```python
from build123d import *

# Parameters (mm, degrees)
F1_DEPTH    = 5
F2_T1_DEPTH = 21.2627511202


# Not quite as in the source:
# - a fillet or chamfer that OpenCascade refuses, or shapes differently, is made with other operations: its cross-section is extruded or revolved along the edge and cut away or added


with BuildPart() as f1:
    # F0 (on Front) → F1 (new body)
    with BuildSketch(Plane.XZ):
        with BuildLine():
            Line((4, -0.5), (5, -0.5))
            ThreePointArc((5, -0.5), (4.7071067812, 0.2071067812), (4, 0.5))
            Line((4, 0.5), (-4, 0.5))
            ThreePointArc((-4, 0.5), (-4.7071067812, 0.2071067812), (-5, -0.5))
            Line((-5, -0.5), (-4, -0.5))
            ThreePointArc((-4, -0.5), (-3.2187502413, -1.2763021336), (-3.625, -2.3))
            Line((-3.625, -2.3), (-2.75, -6.5))
            Line((-2.75, -6.5), (0, -6.5))
            Line((0, -6.5), (2.75, -6.5))
            Line((2.75, -6.5), (3.625, -2.3))
            ThreePointArc((3.625, -2.3), (3.2187502413, -1.2763021336), (4, -0.5))
        make_face()
    extrude(amount=F1_DEPTH)

    # F2: fillet of radius 4 on 2 edges, made by hand

    # F2_s2 → F2_t1 (cut)
    with BuildSketch(Plane.XZ.offset(-8.1313755601)):
        with BuildLine():
            ThreePointArc((0.502550224, -6.5), (-2.0210119343, -5.6034873985), (-3.4133714549, -3.3158170164))
            Line((-3.4133714549, -3.3158170164), (-2.75, -6.5))
            Line((-2.75, -6.5), (0.502550224, -6.5))
        make_face()
        with BuildLine():
            ThreePointArc((3.4133714549, -3.3158170164), (2.0210119343, -5.6034873985), (-0.502550224, -6.5))
            Line((-0.502550224, -6.5), (2.75, -6.5))
            Line((2.75, -6.5), (3.4133714549, -3.3158170164))
        make_face()
    extrude(amount=F2_T1_DEPTH, mode=Mode.SUBTRACT)


solid = f1.part
```
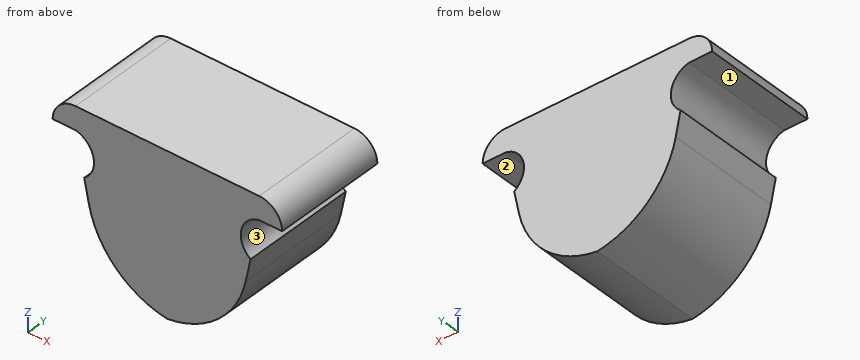
Input: part model. Units: mm. Frame: model coordinates. Face numbers are marked on the shaded views. A direction names the side the tool comes from. Give positions to 0.01 mm unless a question says otherwise; leave off trailing zeros. Order: outer loops, then holes, each group sorted by start corner. A loop starts at its lowest first (then second) coordinate and runs counter-clockwise, first axis right, second up.
1. Section B-B on x = -3. Return the cut outline in (y, z), and give its area (3 significant figures).
Derived:
outline: (-5, -4.43) - (0, -4.43) - (0, 0.5) - (-5, 0.5) - close
area: 24.7 mm2
2. Reachability of the marked faces 1, 2 and 3 from +Z, -Z, +X, -X, +Y, -Y: full face, straight path, thin tool, end or side. Return the list, or none.
Derived:
face 1: -Z, -X, +Y, -Y
face 2: -Z, +X, +Y, -Y
face 3: +X, +Y, -Y
3. Material intervals for L1, parallel to Z at x = -4, y = -1.55; L2, parallel to X at y = -4, z = -1.5; L3, parallel to Z at x = 4.5, y = -0.7, sorted ascending.
Derived:
L1: z = -0.5 to 0.5
L2: x = -3.2 to 3.2
L3: z = -0.5 to 0.37
4. Section A-A on y = -3.8. Return the cut outline in (x, z) (3 decimals).
Derived:
outline: (-5, -0.5) - (-4, -0.5) arc R1 cw to (-3.625, -2.3) - (-3.413, -3.316) arc R4 ccw to (0, -6.468) arc R4 ccw to (3.413, -3.316) - (3.625, -2.3) arc R1 cw to (4, -0.5) - (5, -0.5) arc R1 ccw to (4, 0.5) - (-4, 0.5) arc R1 ccw to start
5. Pin query (flat end, axial travel): pin 1 (2 mm diameter, centred on y = -2.5, z = -2, fed in from -X) (3 decimals); pin 2 (2 mm diameter, centred on y = -3, z = -5, fed in from +X); pin 3 (0.5 mm diameter, centred on x = -4.5, y = -2, fed in from -Z). Return the tip coordinate at first contact, or that it passes through.
Derived:
pin 1: stops at x = -3.625
pin 2: stops at x = 3.21
pin 3: stops at z = -0.5
6. Section C-C on z = -2. Return the cut outline in (x, y).
Derived:
outline: (-3.34, -5) - (3.34, -5) - (3.34, 0) - (-3.34, 0) - close
